Answer from the drawing. Dimensions are ordinates in mm from the lowest x, y and z of the part. Give positions to 0.01 mm unless a question says otherwise; leave off trailing zeros. Order: outer loops, then holes, each group sorted by start corner. A loop starts at its lowest first (then second) coordinate and runs counter-clockwise, first axis right, second up. Notation, with made-up numbers: (-30.5, 6.5) - (-5.5, 6.5) arc R22 cw to (-5.5, 19.5) - close; hole circle Ø1 at (70.25, 40.5). An arc over 180 degrees is marked (long way). Answer in a Markdown table with one row per item.
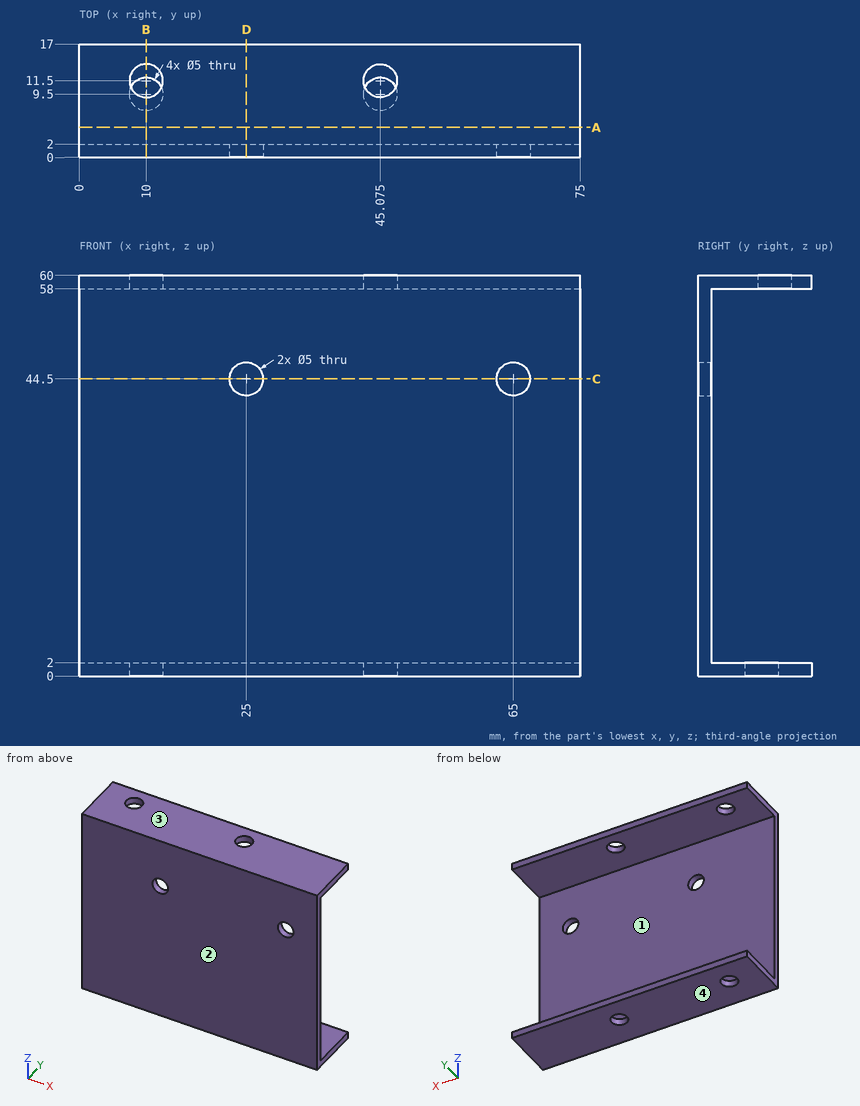
Item 1: Find section B-B on x = 10. Write down the section's boundary in (y, z), then the cut area to 3 significant figures.
Answer block:
| item | result |
|---|---|
| outline | (0, 0) - (7, 0) - (7, 2) - (2, 2) - (2, 58) - (9, 58) - (9, 60) - (0, 60) - close; (12, 0) - (17, 0) - (17, 2) - (12, 2) - close; (14, 58) - (17, 58) - (17, 60) - (14, 60) - close |
| area | 160 mm² |
Item 2: Each of these flat-tipped pins is pushed along its axis until it touches: P1, Ø3, axis at x = 45.075, y = 9.5, coming from the -Z side; P2, Ø1, axis at x = 41.5, z = 31, coming from the +Y side. Where does it stop, or does it pass through?
Answer block:
| item | result |
|---|---|
| P1 | z = 58 |
| P2 | y = 2 |
Item 3: Find section A-A on y = 4.5. Write down the section's boundary in (x, z).
Answer block:
| item | result |
|---|---|
| outline | (0, 0) - (75, 0) - (75, 2) - (0, 2) - close; (0, 58) - (75, 58) - (75, 60) - (0, 60) - close |
Item 4: Determine the mould class of the marked faces 1, 2, 3 and 4 for opening direction Z: pulls with the +Z half, pulls with the -Z half, needs draft (parallel to the pull), parting line crosses it, or undercut.
Answer block:
| item | result |
|---|---|
| face 1 | undercut |
| face 2 | needs draft |
| face 3 | pulls with the +Z half |
| face 4 | pulls with the -Z half |
Item 5: Consider line 1 (Z direction, x = 49.5, y = 13); line 2 (Y direction, x = 10, z = 59); line 3 (X direction, y = 0.6, z = 44.5). Determine where each line is inside the solid, lowest interval first.
Answer block:
| item | result |
|---|---|
| line 1 | 0 to 2, 58 to 60 |
| line 2 | 0 to 9, 14 to 17 |
| line 3 | 0 to 22.5, 27.5 to 62.5, 67.5 to 75 |
Item 6: Find section C-C on z = 44.5. Write down the section's boundary in (x, y).
Answer block:
| item | result |
|---|---|
| outline | (0, 0) - (22.5, 0) - (22.5, 2) - (0, 2) - close; (27.5, 0) - (62.5, 0) - (62.5, 2) - (27.5, 2) - close; (67.5, 0) - (75, 0) - (75, 2) - (67.5, 2) - close |
Item 7: Find section D-D on x = 25. Write down the section's boundary in (y, z).
Answer block:
| item | result |
|---|---|
| outline | (0, 0) - (17, 0) - (17, 2) - (2, 2) - (2, 42) - (0, 42) - close; (0, 47) - (2, 47) - (2, 58) - (17, 58) - (17, 60) - (0, 60) - close |
